CAD build for the part. Positions are in the model's coordinates, mm. A direction names the side the tool comes from. Give positions to 0.01 mm unless a question says otherwise; leave off trailing zeros. Order: outer loops, then holes, each group sorted by start corner. A loop starts at its lowest first (then second) coordinate and runs counter-clockwise, first axis right, second up.
from build123d import *

# Parameters (mm, degrees)
SKETCH_1_W          = 15
SKETCH_1_H          = 100
EXTRUDE_1_DEPTH     = 15
SKETCH_3_W          = 10.35
SKETCH_3_H          = 10.35
SKETCH_3_W_2        = 10.4
SKETCH_3_H_2        = 10.4
SKETCH_3_W_3        = 10.45
SKETCH_3_H_3        = 10.45
SKETCH_3_W_4        = 10.5
SKETCH_3_H_4        = 10.5
CUT_EXTRUDE_1_DEPTH = 10
SKETCH_4_W          = 15
SKETCH_4_H          = 12.316827503
CUT_EXTRUDE_2_DEPTH = 53.737557774


with BuildPart() as part:
    # 草图1 → 凸台-拉伸1 (new body)
    with BuildSketch(Plane.XY):
        Rectangle(SKETCH_1_W, SKETCH_1_H)
    extrude(amount=EXTRUDE_1_DEPTH)

    # 草图3 → 切除-拉伸1 (cut)
    with BuildSketch(Plane.XY.offset(15)):
        with Locations((0, 26.925)):
            Rectangle(SKETCH_3_W, SKETCH_3_H)
        with Locations((0, 10.55)):
            Rectangle(SKETCH_3_W_2, SKETCH_3_H_2)
        with Locations((0, -5.875)):
            Rectangle(SKETCH_3_W_3, SKETCH_3_H_3)
        with Locations((0, -22.3)):
            Rectangle(SKETCH_3_W_2, SKETCH_3_H_2)
        with Locations((0, -38.75)):
            Rectangle(SKETCH_3_W_4, SKETCH_3_H_4)
    extrude(amount=-CUT_EXTRUDE_1_DEPTH, mode=Mode.SUBTRACT)

    # 草图4 → 切除-拉伸2 (cut, through all)
    with BuildSketch(Plane.XY.offset(15)):
        with Locations((0, 43.841586249)):
            Rectangle(SKETCH_4_W, SKETCH_4_H)
    extrude(amount=-CUT_EXTRUDE_2_DEPTH, mode=Mode.SUBTRACT)


solid = part.part
1. Mould opens along Y. For faces 1 (the flat face through (7.5, -7, 7)), 2 (the flat face through (0, -17.1, 10)), 3 (the flat face through (0, 37.683, 8)) say: released by +Y, released by -Y, zero draft, split by the parting line, or undercut.
2. Saw through at A-A on z = 8.25. Give the cut face in (x, y) (3 decimals), plus the area to 3 significant figures.
3. Wall check: line 1 (Y direction, x = 1.5, z = 7.5); line 2 (X direction, y = 27, z = 6.75) (3 decimals); line 3 (Z direction, x = -3.75, y = 27). Give the ranges that are in metal, low to high.
4. Saw through at B-B on x = 3.75. Give the cut face in (y, z).
5. Saw through at C-C on y = -26. Give the cut face in (x, z), plus the area to 3 significant figures.
6. Saw through at D-D on y = 25. Give the cut face in (x, z) (3 decimals).
7. Pin check, flat tip, straight feed: P1, Ø3, axis at x = 2, y = 13, coming from the +Z side. Stop position of the tip, or through.
8. 3-axis set-ups, long thin cutter, end or side, ignore diameter. For faces 4 (the flat face through (0, -50, 7)), 5 (the flat face through (0, -39, 5)): which of +Z, -Z, +X, -X, +Y, -Y reach the whole face in a straight line?
Reported:
1. face 1: zero draft
1. face 2: undercut
1. face 3: released by +Y
2. outline: (-7.5, -50) - (7.5, -50) - (7.5, 37.683) - (-7.5, 37.683) - close; hole (-5.25, -44) - (5.25, -44) - (5.25, -33.5) - (-5.25, -33.5) - close; hole (-5.225, -11.1) - (5.225, -11.1) - (5.225, -0.65) - (-5.225, -0.65) - close; hole (-5.2, -27.5) - (5.2, -27.5) - (5.2, -17.1) - (-5.2, -17.1) - close; hole (-5.2, 5.35) - (5.2, 5.35) - (5.2, 15.75) - (-5.2, 15.75) - close; hole (-5.175, 21.75) - (5.175, 21.75) - (5.175, 32.1) - (-5.175, 32.1) - close
2. area: 772 mm2
3. line 1: y = -50 to -44, -33.5 to -27.5, -17.1 to -11.1, -0.65 to 5.35, 15.75 to 21.75, 32.1 to 37.68
3. line 2: x = -7.5 to -5.175, 5.175 to 7.5
3. line 3: z = 0 to 5
4. outline: (-50, 0) - (37.68, 0) - (37.68, 15) - (32.1, 15) - (32.1, 5) - (21.75, 5) - (21.75, 15) - (15.75, 15) - (15.75, 5) - (5.35, 5) - (5.35, 15) - (-0.65, 15) - (-0.65, 5) - (-11.1, 5) - (-11.1, 15) - (-17.1, 15) - (-17.1, 5) - (-27.5, 5) - (-27.5, 15) - (-33.5, 15) - (-33.5, 5) - (-44, 5) - (-44, 15) - (-50, 15) - close
5. outline: (-7.5, 0) - (7.5, 0) - (7.5, 15) - (5.2, 15) - (5.2, 5) - (-5.2, 5) - (-5.2, 15) - (-7.5, 15) - close
5. area: 121 mm2
6. outline: (-7.5, 0) - (7.5, 0) - (7.5, 15) - (5.175, 15) - (5.175, 5) - (-5.175, 5) - (-5.175, 15) - (-7.5, 15) - close
7. P1: stops at z = 5
8. face 4: +Z, -Z, +X, -X, -Y
8. face 5: +Z
